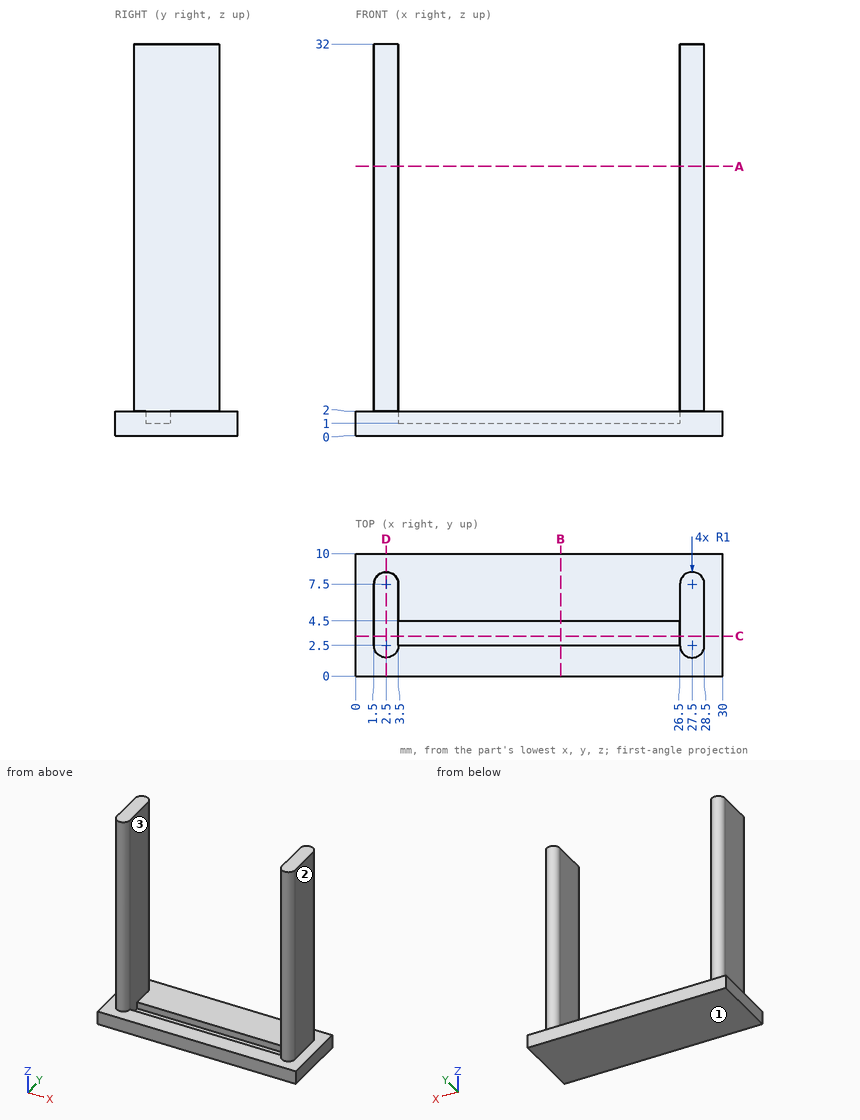
Drawing for the job (mm, zero at the part's lowest x, y, z). Give positions to 0.01 mm unless a question says otherwise; leave off trailing zeros. Loops run counter-clockwise (first coordinate to the right, second up) from the corner with the lowest first, then second, coordinate; pieces in that order, holes last. Notation, with made-up numbers: (-3.75, -7) - (18.25, -7) arc R10 cw to (18.25, 2) - close; hole circle Ø8 at (52, 43). An arc over 180 degrees is marked (long way). Write item = value, one per line. Start each with the question number.
1) Band-saw the part on B-B on x = 16.75. Give the cut face in (y, z).
2) Band-saw the part on A-A on z = 22. Give the cut face in (x, y).
3) Band-saw the part on C-C on y = 3.25. Give the cut face in (x, z).
4) Band-saw the part on D-D on x = 2.5. Give the cut face in (y, z).
5) Pull direction X, two halves, no side cores. Call the marked faces 1, 2 and 3: +X half, -X half, draft (parallel to the pull), parting line (faces both ways), or undercut.
6) Drop flat-ended pins along their axis: pin 1 Ø4 at (y, z) = (6.5, 26) entering from +X; pin 2 Ø1.5 at (y, z) = (1.5, 12) entering from -X; pin 3 Ø1.6 at (x, y) = (16.5, 4) entering from +Z. Give the stop position or say it passes through.
7) Probe probe 1 along X at (y, z) = (3.25, 21.5); probe 2 along Z at (x, y) = (12.25, 9.25); probe 3 along Z at (x, y) = (6.75, 3). List the from-to ranges inside material, lowest first. Write a range as from..to.
Final values:
q1.outline = (0, 0) - (10, 0) - (10, 2) - (4.5, 2) - (4.5, 1) - (2.5, 1) - (2.5, 2) - (0, 2) - close
q2.outline = (1.5, 2.5) arc R1 ccw to (3.5, 2.5) - (3.5, 7.5) arc R1 ccw to (1.5, 7.5) - close; (26.5, 2.5) arc R1 ccw to (28.5, 2.5) - (28.5, 7.5) arc R1 ccw to (26.5, 7.5) - close
q3.outline = (0, 0) - (30, 0) - (30, 2) - (28.5, 2) - (28.5, 32) - (26.5, 32) - (26.5, 1) - (3.5, 1) - (3.5, 32) - (1.5, 32) - (1.5, 2) - (0, 2) - close
q4.outline = (0, 0) - (10, 0) - (10, 2) - (8.5, 2) - (8.5, 32) - (1.5, 32) - (1.5, 2) - (0, 2) - close
q5.face_1 = draft
q5.face_2 = +X half
q5.face_3 = undercut
q6.pin_1 = 28.5
q6.pin_2 = 1.53
q6.pin_3 = 2
q7.probe_1 = 1.5..3.5, 26.5..28.5
q7.probe_2 = 0..2
q7.probe_3 = 0..1
